```python
from build123d import *

# Parameters (mm, degrees)
SKETCH1_W           = 76.2
SKETCH1_H           = 25.4
BOSS_EXTRUDE1_DEPTH = 12.7
CUT_EXTRUDE1_DEPTH  = 13.7
SKETCH4_W           = 6.35
SKETCH4_H           = 4.572
SKETCH4_H_2         = 2.286
CUT_EXTRUDE2_DEPTH  = 26.4


with BuildPart() as part:
    # Sketch1 → Boss-Extrude1 (new body)
    with BuildSketch(Plane(origin=(0, 0, 0), x_dir=(1, 0, 0), z_dir=(0, 1, 0))):
        with Locations((38.1, 12.7)):
            Rectangle(SKETCH1_W, SKETCH1_H)
    extrude(amount=BOSS_EXTRUDE1_DEPTH)

    # Sketch3 → Cut-Extrude1 (cut, through all)
    with BuildSketch(Plane(origin=(0, 12.7, 0), x_dir=(1, 0, 0), z_dir=(0, 1, 0))):
        with BuildLine():
            Line((15.875, 8.5725), (60.325, 8.5725))
            ThreePointArc((60.325, 8.5725), (62.57006403, 9.50243597), (63.5, 11.7475))
            Line((63.5, 11.7475), (63.5, 13.6525))
            ThreePointArc((63.5, 13.6525), (62.57006403, 15.89756403), (60.325, 16.8275))
            Line((60.325, 16.8275), (15.875, 16.8275))
            ThreePointArc((15.875, 16.8275), (13.62993597, 15.89756403), (12.7, 13.6525))
            Line((12.7, 13.6525), (12.7, 11.7475))
            ThreePointArc((12.7, 11.7475), (13.62993597, 9.50243597), (15.875, 8.5725))
        make_face()
    extrude(amount=-CUT_EXTRUDE1_DEPTH, mode=Mode.SUBTRACT)

    # Sketch4 → Cut-Extrude2 (cut, through all)
    with BuildSketch(Plane.XY):
        with Locations((3.175, 2.286)):
            Rectangle(SKETCH4_W, SKETCH4_H)
        with Locations((3.175, 11.557)):
            Rectangle(SKETCH4_W, SKETCH4_H_2)
    extrude(amount=-CUT_EXTRUDE2_DEPTH, mode=Mode.SUBTRACT)


solid = part.part
```
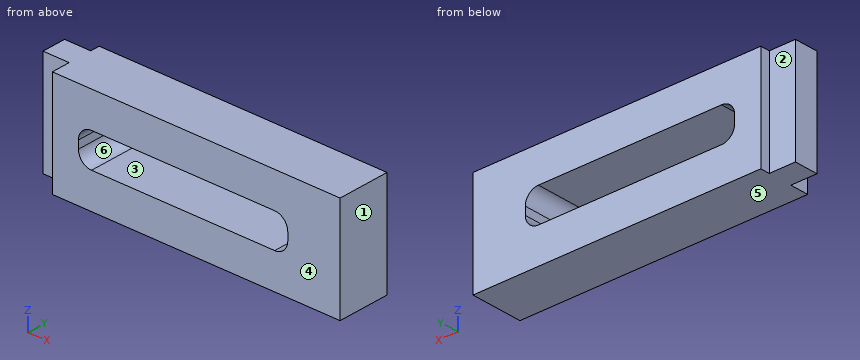
Read the model definition and answer for the solid it produces. Units are mm, in the model's axes. Face numbers are marked on the shaded views. A direction names the side the tool comes from. Give positions to 0.01 mm unless a question says otherwise; leave off trailing zeros. Loops run counter-clockwise (first coordinate to the right, second up) from the corner with the lowest first, then second, coordinate; pieces in that order, holes last.
Item 1: The part is cut by section C-C (z = -4.75). Write down the section's boundary in (x, y).
Item 2: The part is cut by section A-A (x = 46). Write down the section's boundary in (y, z), and give its area (3 significant figures).
Item 3: Each of these flat-tipped pins is pushed along its axis until it touches: pin 1 Ø1.4 at (y, z) = (2, -15) entering from -X; pin 2 Ø7 at (x, z) = (2, -11.5) entering from +Y; pin 3 Ø5 at (x, z) = (2.5, -9.5) entering from -Y. Where does it stop, or does it pass through?
Item 4: The mould has two halves that part along Z. Classify the marked faces 4, 5 and 6: released by +Z, released by -Z, zero draft, split by the parting line, or undercut.
Item 5: Find the intervals of material crossed by line 1 along Z through (x, y) = (19, 10.25); line 2 along X through (y, z) = (9.25, -11.5); line 3 along X through (y, z) = (1, -20.5), in increasing order.
Item 6: For the marked faces 1, 2 and 3, determine the directions among +Z, -Z, +X, -X, +Y, -Y from which every point of the face is accessible in a straight line to the end or side of a thin tool.
Item 7: The part is cut by section D-D (z = -10.5). Write down the section's boundary in (x, y).
Taken from the geometry:
1. outline: (0, 4.57) - (6.35, 4.57) - (6.35, 0) - (76.2, 0) - (76.2, 12.7) - (6.35, 12.7) - (6.35, 10.41) - (0, 10.41) - close
2. outline: (0, -25.4) - (12.7, -25.4) - (12.7, -16.83) - (0, -16.83) - close; (0, -8.57) - (12.7, -8.57) - (12.7, 0) - (0, 0) - close
2. area: 218 mm2
3. pin 1: stops at x = 6.35
3. pin 2: stops at y = 10.41
3. pin 3: stops at y = 4.57
4. face 4: zero draft
4. face 5: released by -Z
4. face 6: undercut
5. line 1: z = -25.4 to -16.83, -8.57 to 0
5. line 2: x = 0 to 12.71, 63.49 to 76.2
5. line 3: x = 6.35 to 76.2
6. face 1: +Z, -Z, +X, +Y, -Y
6. face 2: +Z, -Z, -X, +Y
6. face 3: +Y, -Y
7. outline: (0, 4.57) - (6.35, 4.57) - (6.35, 0) - (12.96, 0) - (12.96, 12.7) - (6.35, 12.7) - (6.35, 10.41) - (0, 10.41) - close; (63.24, 0) - (76.2, 0) - (76.2, 12.7) - (63.24, 12.7) - close
